Verification items for the finished model (mm, model axes). Face numbers are marked on the shaded views. A direction names the side the tool comes from. Give positions to 0.01 mm unless a question says otherwise; leave off trailing zeros. Write each loop counter-clockwise with the first axis right and the second up, starting at its lowest first coordinate (ties: lowest second). Pieces come first, ordered by that corner, then holes. Notation, with made-up numbers: (84, 42) - (99, 42) arc R19 ccw to (99, 46) - close; hole circle Ø3 at (21.25, 47). An arc over 180 degrees is marked (long way). Answer as a JSON object with one key per item and string values. Group by question number.
Item 1: Sectioned sample at D-D, the plane x = -4. Record the boundary of the cut face in (y, z).
Item 2: Tool access check on the marked faces 1, 2, 3 and 4. Record the directions out of +Z, -Z, +X, -X, +Y, -Y that give a thin tool (end or side, any length) a straight path to the whole face; none if there is none.
Item 3: Go/stop test with flat-tipped pins: pin 1 (0.8 mm diameter, centred on y = 1, z = 3.5, fed in from -X); pin 2 (4.5 mm diameter, centred on x = -30.5, y = -0.5, fed in from +Z); pin 3 (2 mm diameter, centred on y = 5.5, z = -4.5, fed in from -X); pin 4 (3 mm diameter, centred on x = -14.5, z = -10, fed in from -Y). Record where each tip stops, or that it passes through.
Item 4: Scan lines: line 1 along Z through (x, y) = (-23, 0); line 2 along Z through (x, y) = (-17.25, 0). Record each from-to range of solid material in increasing order. Write a range as [from, to].
Item 5: Sectioned sample at C-C, the plane x = -13. Record the boundary of the cut face in (y, z), and give its area (3 significant figures).
Item 6: Sectioned sample at A-A, the plane z = 0. Record the boundary of the cut face in (x, y), and give its area (3 significant figures).
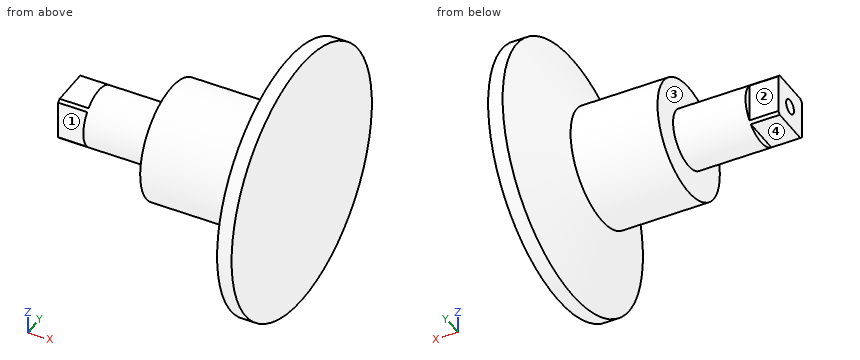
```python
from build123d import *

# Parameters (mm, degrees)
F2_R     = 1
F3_DEPTH = 4


with BuildPart() as f1:
    # F0 (on Front) → F1 (revolve)
    with BuildSketch(Plane.XZ):
        Polygon((-6, 8), (-18, 8), (-18, 4), (-32, 4), (-32, 1), (-12, 1), (-12, 0), (0, 0), (0, 18), (-2, 18), align=None)
    revolve(axis=Axis((0, 0, 0), (1, 0, 0)))

    # F2 (on face) → F3 (cut)
    with BuildSketch(Plane(origin=(-32, 0, 0), x_dir=(0, -1, 0), z_dir=(-1, 0, 0))):
        Circle(F2_R)
        with BuildLine():
            ThreePointArc((2.6457513111, 3), (0, 4), (-2.6457513111, 3))
            Line((-2.6457513111, 3), (2.6457513111, 3))
        make_face()
        with BuildLine():
            ThreePointArc((4, 0), (3.7416573868, 1.4142135624), (3, 2.6457513111))
            Line((3, 2.6457513111), (3, -2.6457513111))
            ThreePointArc((3, -2.6457513111), (3.7416573868, -1.4142135624), (4, 0))
        make_face()
        with BuildLine():
            Line((2.6457513111, -3), (-2.6457513111, -3))
            ThreePointArc((-2.6457513111, -3), (0, -4), (2.6457513111, -3))
        make_face()
        with BuildLine():
            Line((-3, -2.6457513111), (-3, 2.6457513111))
            ThreePointArc((-3, 2.6457513111), (-4, 0), (-3, -2.6457513111))
        make_face()
    extrude(amount=-F3_DEPTH, mode=Mode.SUBTRACT)


solid = f1.part
```
Geometry check:
{
 "1": {"outline": "circle Ø26 at (0, 0)"},
 "2": {"face 1": "+Z, -Z, -X, -Y", "face 2": "+Z, -Z, -X, +Y", "face 3": "-X", "face 4": "-Z, -X, +Y, -Y"},
 "3": {"pin 1": "x = -28", "pin 2": "z = 3", "pin 3": "x = -18", "pin 4": "through"},
 "4": {"line 1": "[-4, -1], [1, 4]", "line 2": "[-8, -1], [1, 8]"},
 "5": {"outline": "circle Ø16 at (0, 0); hole circle Ø2 at (0, 0)", "area": "198 mm^2"},
 "6": {"outline": "(-32, -3) - (-28, -3) - (-28, -4) - (-18, -4) - (-18, -8) - (-6, -8) - (-2, -18) - (0, -18) - (0, 18) - (-2, 18) - (-6, 8) - (-18, 8) - (-18, 4) - (-28, 4) - (-28, 3) - (-32, 3) - (-32, 1) - (-12, 1) - (-12, -1) - (-32, -1) - close", "area": "432 mm^2"}
}
